Input: part model. Units: mm. Frame: model coordinates. A direction names the side the tool comes from. Round coordinates to 2 decimals unless told otherwise and drop trailing zeros. Order: outer loops, then holes, each group sorted by start corner. A loop starts at its lowest first (then second) coordinate and runs counter-clockwise, first axis right, second up.
Item 1: Line query: L1, parallel to X at y = 0, z = -2.75; L2, parallel to Z at x = -142.5, y = 8.25; L3, parallel to X at y = 0, z = -7.25. Output: solid intervals per line, ascending.
Item 2: Cut plane B-B on z = -28. Output: boundary loops of the cut face in (x, y).
Item 3: Cut plane A-A on y = 0. Output: boundary loops of the cut face in (x, z), then the cut area to 3 significant figures.
Item 4: First-contact query: pin 1 (10 mm diameter, centred on x = 77, z = -117.5, fed in from +Y); pin 2 (4 mm diameter, centred on y = 0, z = -112.5, fed in from +X); pin 3 (12.5 mm diameter, centred on x = -154, y = -1, fed in from -Z); pin 4 (13.5 mm diameter, centred on x = 150.52, y = 0, fed in from -Z). Flat tips, straight axial feed; report the tip coordinate or a pass-through.
Item 5: Mould query, pull axis X, two halves, no side actions, for faces 3 (the flat face through (151, -6, -11.341)), 4 (the flat face through (163.5, 0, -6)), 5 (the cylindrical face through (-156.013, -3.302, -6.084)), 6 (the cylindrical face through (154.548, -1.269, -5.75)). Classes: released by +X, released by -X, zero draft, split by the parting line, or undercut.
Item 6: Cut plane C-C on x = 0. Output: boundary loops of the cut face in (y, z), then the cut area to 3 significant figures.
Item 7: Cut plane D-D on z = -71. Output: boundary loops of the cut face in (x, y).
Item 8: Reachability of faces 1 (the flat face through (-138, 0, 0)), 2 (the flat face through (-148, -3, -12)) from +Z, -Z, +X, -X, +Y, -Y: full face, straight path, thin tool, end or side. Return the list, or none.
```python
from build123d import *

# Parameters (mm, degrees)
F1_DEPTH = 12.5
F2_R     = 4.225259
F3_DEPTH = 11.342264
F4_R     = 4.884984
F5_DEPTH = 25


with BuildPart() as f1:
    # F0 (on Front) → F1 (new body, symmetric)
    with BuildSketch(Plane.XZ):
        with BuildLine():
            ThreePointArc((113.5, 0), (0, -113.5), (-113.5, 0))
            Line((-113.5, 0), (-138.5, 0))
            Line((-138.5, 0), (-163.5, 0))
            Line((-163.5, 0), (-163.5, -12))
            Line((-163.5, -12), (-137.979165, -12))
            ThreePointArc((-137.979165, -12), (0.330544, -138.499606), (138.034871, -11.341264))
            Line((138.034871, -11.341264), (163.5, -11.341264))
            Line((163.5, -11.341264), (163.5, 0))
            Line((163.5, 0), (138.5, 0))
            Line((138.5, 0), (113.5, 0))
        make_face()
    extrude(amount=F1_DEPTH, both=True)

    # F2 (on face) → F3 (cut, through all)
    with BuildSketch(Plane(origin=(0, 0, -11.341264), x_dir=(1, 0, 0), z_dir=(0, 0, -1))):
        with Locations((150.517523, 0)):
            Circle(F2_R)
    extrude(amount=-F3_DEPTH, mode=Mode.SUBTRACT)

    # F4 (on face) → F5 (cut)
    with BuildSketch(Plane(origin=(0, 0, -12), x_dir=(1, 0, 0), z_dir=(0, 0, -1))):
        with Locations((-152.41228, 0)):
            Circle(F4_R)
    extrude(amount=-F5_DEPTH, mode=Mode.SUBTRACT)


solid = f1.part
```
From the geometry:
1. L1: x = -163.5 to -157.3, -147.53 to -113.47, 113.47 to 146.29, 154.74 to 163.5
1. L2: z = -12 to 0
1. L3: x = -163.5 to -157.3, -147.53 to -113.27, 113.27 to 146.29, 154.74 to 163.5
2. outline: (-135.64, -12.5) - (-109.99, -12.5) - (-109.99, 12.5) - (-135.64, 12.5) - close; (109.99, -12.5) - (135.64, -12.5) - (135.64, 12.5) - (109.99, 12.5) - close
3. outline: (-163.5, -12) - (-157.3, -12) - (-157.3, 0) - (-163.5, 0) - close; (-147.53, -12) - (-137.98, -12) arc R138.5 ccw to (138.03, -11.34) - (146.29, -11.34) - (146.29, 0) - (113.5, 0) arc R113.5 cw to (-113.5, 0) - (-147.53, 0) - close; (154.74, -11.34) - (163.5, -11.34) - (163.5, 0) - (154.74, 0) - close
3. area: 10,300 mm2
4. pin 1: stops at y = 12.5
4. pin 2: stops at x = 83.5
4. pin 3: stops at z = -12
4. pin 4: stops at z = -11.34
5. face 3: zero draft
5. face 4: released by +X
5. face 5: undercut
5. face 6: undercut
6. outline: (-12.5, -138.5) - (12.5, -138.5) - (12.5, -113.5) - (-12.5, -113.5) - close
6. area: 625 mm2
7. outline: (-118.92, -12.5) - (-88.55, -12.5) - (-88.55, 12.5) - (-118.92, 12.5) - close; (88.55, -12.5) - (118.92, -12.5) - (118.92, 12.5) - (88.55, 12.5) - close
8. face 1: +Z, +X, -X, +Y, -Y
8. face 2: -Z, -X, +Y, -Y
